from build123d import *

# Parameters (mm, degrees)
SKETCH1_W           = 17
SKETCH1_H           = 45
BOSS_EXTRUDE1_DEPTH = 50
CUT_EXTRUDE1_DEPTH  = 68.803023531
CUT_EXTRUDE3_DEPTH  = 50.350151975


with BuildPart() as part:
    # Sketch1 → Boss-Extrude1 (new body)
    with BuildSketch(Plane(origin=(0, 0, 0), x_dir=(1, 0, 0), z_dir=(0, 1, 0))):
        Rectangle(SKETCH1_W, SKETCH1_H)
    extrude(amount=BOSS_EXTRUDE1_DEPTH)

    # Sketch2 → Cut-Extrude1 (cut, through all)
    with BuildSketch(Plane.XY.offset(22.5)):
        Polygon((8.5, 50), (-8.5, 40.185045424), (-8.5, 50), align=None)
    extrude(amount=-CUT_EXTRUDE1_DEPTH, mode=Mode.SUBTRACT)

    # Sketch3 → Cut-Extrude3 (cut, through all)
    with BuildSketch(Plane(origin=(-19.525635095, 33.819392034, 0), x_dir=(0.8660254037844417, 0.4999999999999949, 0), z_dir=(-0.4999999999999949, 0.8660254037844417, 0))):
        Polygon((25.078911087, -18.5), (19.078911087, -18.5), (19.078911087, -10.994373166), (12.73130678, 0), (19.078911087, 10.994373166), (19.078911087, 18.5), (25.078911087, 18.5), (25.078911087, 16), (40.444119701, 16), (49.681724008, 0), (40.444119701, -16), (25.078911087, -16), align=None)
    extrude(amount=-CUT_EXTRUDE3_DEPTH, mode=Mode.SUBTRACT)


solid = part.part
Design review of the part built by this model. Coordinates are the model's own, in mm. A direction names the side the tool comes from. Give positions to 0.01 mm unless a question says otherwise; leave off trailing zeros. Loops run counter-clockwise (first coordinate to the right, second up) from the corner with the lowest first, then second, coordinate; pieces in that order, holes last. Notation, with made-up numbers: (16, 39) - (58, 39) arc R30 cw to (58, 67) - close; hole circle Ø9 at (-6, 31). An arc over 180 degrees is marked (long way). Write item = value, one per line.
1) To check wall thickness, follow line 1 (Z direction, x = 2, y = 36.5); line 2 (Z direction, x = 5.5, y = 42); line 3 (Y direction, x = 5.25, z = -18). State the ranges of each line that lie inside material, in increasing order.
Result sheet:
line_1 = -22.5 to -18.5, 18.5 to 22.5
line_2 = -22.5 to -16, 16 to 22.5
line_3 = 0 to 29.06, 41.06 to 48.12
2) Take a section at D-D on y = 39. State the section outline as (x, z) points.
Result sheet:
outline = (-8.5, -22.5) - (8.5, -22.5) - (8.5, -16) - (6.44, -16) - (6.44, -18.5) - (-0.49, -18.5) - (-0.49, -10.99) - (-7.82, 0) - (-0.49, 10.99) - (-0.49, 18.5) - (6.44, 18.5) - (6.44, 16) - (8.5, 16) - (8.5, 22.5) - (-8.5, 22.5) - close
3) Take a section at A-A on z = -12. State the section outline as (x, y) points, and give its area (3 significant figures).
Result sheet:
outline = (-8.5, 0) - (8.5, 0) - (8.5, 23.44) - (-3, 43.36) - (-8.5, 40.19) - close
area = 614 mm2
4) Take a section at B-B on y = 45.5. State the section outline as (x, z) points.
Result sheet:
outline = (0.71, -22.5) - (8.5, -22.5) - (8.5, -16) - (2.69, -16) - (2.69, -18.5) - (0.71, -18.5) - close; (0.71, 18.5) - (2.69, 18.5) - (2.69, 16) - (8.5, 16) - (8.5, 22.5) - (0.71, 22.5) - close
5) Take a section at C-C on x = -1.5. State the section outline as (y, z) points, and give its area (3 significant figures).
Result sheet:
outline = (0, -22.5) - (44.23, -22.5) - (44.23, -18.5) - (40.76, -18.5) - (40.76, -10.99) - (28.06, 0) - (40.76, 10.99) - (40.76, 18.5) - (44.23, 18.5) - (44.23, 22.5) - (0, 22.5) - close
area = 1,720 mm2
6) Draft analysis for pull direction X (two halves, no side actions). For faces 1 (the face through (5.303, 40.974, -17.268)), 2 (the face through (8.5, 14, -5)), 3 (the face through (7, 44, -16)), state which applies: +X half, -X half, draft (parallel to the pull), parting line (faces both ways), or undercut.
Result sheet:
face_1 = undercut
face_2 = +X half
face_3 = draft
7) Tool access review of faces 4 (the face through (0.779, 30.549, 5.574)), 5 (the face through (4, 37, 18.5)), 6 (the face through (-3.66, 42.98, -16.09)): name each direction out of +Z, -Z, +X, -X, +Y, -Y from which nothing blocks a thin tool from reaching the whole face with its end or side.
Result sheet:
face_4 = +X, +Y
face_5 = none
face_6 = +Z, -Z, -X, +Y
8) Clearance check with a flat-ended pin moving along its axis: pin 1 Ø8 at (x, z) = (0.5, 0) entering from +Y. State where the tip first meets the part, or that it passes through.
Result sheet:
pin_1 = 32.92
